```python
from build123d import *

# Parameters (mm, degrees)
SKETCH1_W           = 110
SKETCH1_H           = 30
BOSS_EXTRUDE1_DEPTH = 10
M6_CLEARANCE_HOLE_D = 6.6


with BuildPart() as part:
    # Sketch1 → Boss-Extrude1 (new body)
    with BuildSketch(Plane.XY):
        with Locations((-14.126560257, 689.486311854)):
            Rectangle(SKETCH1_W, SKETCH1_H)
    extrude(amount=BOSS_EXTRUDE1_DEPTH)

    # M6 Clearance Hole (through all)
    with Locations(Plane(origin=(545.719230148, 1586.957920749, 10), x_dir=(-1, 0, 0), z_dir=(0, 0, 1))):
        with Locations((514.845790405, 1450.886073068), (514.845790405, 1412.886073068), (537.845790405, 1453.886073068), (537.845790405, 1409.886073068), (581.845790405, 1453.886073068), (581.845790405, 1409.886073068), (604.845790405, 1450.886073068), (604.845790405, 1412.886073068), (514.845790405, 897.471608895), (537.845790405, 897.471608895), (581.845790405, 897.471608895), (604.845790405, 897.471608895), (394.752371414, 1482.156083565), (514.845790405, 1431.886073068), (537.845790405, 1431.886073068), (581.845790405, 1431.886073068), (604.845790405, 1431.886073068)):
            Hole(M6_CLEARANCE_HOLE_D / 2)


solid = part.part
```
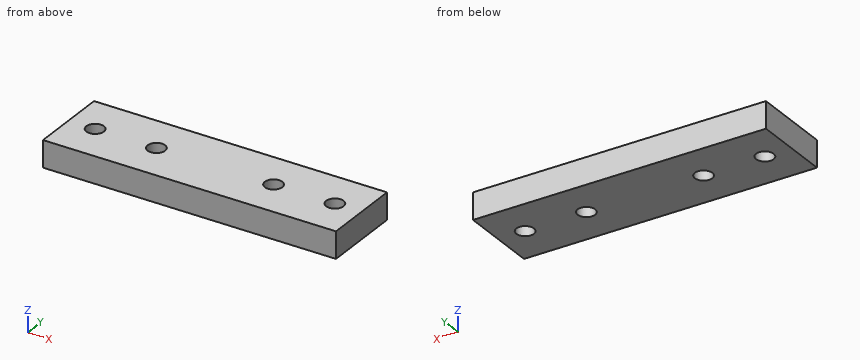
Here's how the part is built. I have some questions about the finished solid (model axes, mm). Coordinates: 2 decimals unless noted, no trailing zeros. Order: outer loops, then holes, each group sorted by start corner. A loop starts at its lowest first (then second) coordinate and runs counter-clockwise, first axis right, second up. Notation, with made-up numbers: M -15.5,40 L 16.5,40 A15 cw 16.5,60 Z; hole C 1,3 d5. An arc over 180 degrees is marked long. Answer as a JSON object with one key per item and string values. Group by question number.
(1) I need wall thicknesses on probe 1 along X at (y, z) = (688.5, 1.75); probe 2 along X at (y, z) = (688, 5.25); probe 3 along Y at (x, z) = (30.5, 5). Which ranges of each line are inside material? Lowest first, please.
(2) Suppose I cut it at C-C, the plane x = -61. Please give me the cut outline in (y, z), then the cut area to 3 significant figures.
(3) Suppose I cut it at A-A, the plane x = 28.5. Please give me the cut outline in (y, z), then the cut area to 3 significant figures.
(4) For pin 1 (8 mm diameter, centred on x = -54.5, y = 697.5, fed in from -Z), with a flat end and sliding along its axis, tell me the tip position at first contact or that it passes through.
(5) Suppose I cut it at B-B, the plane z = 6.5. Please give me the cut outline in (x, y), then the cut area to 3 significant figures.
Values found:
{
 "1": {"probe 1": "x = -69.13 to -62.28, -55.98 to -39.28, -32.98 to 4.72, 11.02 to 27.72, 34.02 to 40.87", "probe 2": "x = -69.13 to -62.07, -56.18 to -39.07, -33.18 to 4.93, 10.82 to 27.93, 33.82 to 40.87", "probe 3": "y = 674.49 to 686.21, 692.77 to 704.49"},
 "2": {"outline": "M 674.49,0 L 686.77,0 L 686.77,10 L 674.49,10 Z; M 692.2,0 L 704.49,0 L 704.49,10 L 692.2,10 Z", "area": "246 mm^2"},
 "3": {"outline": "M 674.49,0 L 687.19,0 L 687.19,10 L 674.49,10 Z; M 691.78,0 L 704.49,0 L 704.49,10 L 691.78,10 Z", "area": "254 mm^2"},
 "4": {"pin 1": "stops at z = 0"},
 "5": {"outline": "M -69.13,674.49 L 40.87,674.49 L 40.87,704.49 L -69.13,704.49 Z; hole C -59.13,689.49 d6.6; hole C -36.13,689.49 d6.6; hole C 7.87,689.49 d6.6; hole C 30.87,689.49 d6.6", "area": "3,160 mm^2"}
}
